Work out the finished part from the listing and answer in its coordinate system (mm). A direction names the side the tool comes from. Give positions to 0.01 mm unless a question says otherwise; leave off trailing zeros. Loops run counter-clockwise (first coordinate to the right, second up) from the corner with the lowest first, then second, coordinate; pieces in that order, holes last. Notation, with made-up numbers: M 9.25,56.25 L 45.25,56.25 A21 cw 45.25,71.25 Z; hole C -37,75.25 d3. An arc over 180 degrees is marked long. Use a Markdown table: item, result.
```python
from build123d import *

# Parameters (mm, degrees)
SKETCH1_W                      = 40.64
SKETCH1_H                      = 2.54
BASE_EXTRUDE_DEPTH             = 5
SKETCH2_W                      = 1.524
SKETCH2_H                      = 0.254
STANDOFF_WIDTH_DEPTH           = 41.966114046
UPPER_START                    = -19.4945
UPPER_CORE_OUTLINE_W           = 3.3528
UPPER_CORE_OUTLINE_H           = 0.889
UPPER_CORE_DEPTH               = 0.889
LEAD_IN_SIZE                   = 0.3937
LEAD_IN_SIZE2                  = 0.469193389
CORE_PATTERN_COUNT             = 16
CORE_PATTERN_PITCH             = 2.54
LEAD_IN_OF_CORE_PATTERN_SIZE2  = 0.469193389
LEAD_IN_OF_CORE_PATTERN_SIZE   = 0.3937
POSITION_CUT_DEPTH             = 21.964620197
SKETCH10_W                     = 0.2794
SKETCH10_H                     = 0.254
STANDOFF_LENGTH_DEPTH          = 22.07970588
STANDOFF_PATTERN_COUNT         = 16
STANDOFF_PATTERN_PITCH         = 2.54
SKETCH11_W                     = 0.635
SKETCH11_H                     = 0.4064
TAIL_DEPTH                     = 3.175
TAIL_FILLETS_R                 = 0.3175
TAIL_PATTERN_COUNT             = 16
TAIL_PATTERN_PITCH             = 2.54
TAIL_FILLETS_OF_TAIL_PATTERN_R = 0.3175
SKETCH12_W                     = 27.94
SKETCH12_H                     = 7.921
CUT_EXTRUDE1_DEPTH             = 22.07970588


# Read off the part's stored shape, not the designer's step: Upper Core
with BuildPart() as part:
    # Sketch1 → Base-Extrude (new body)
    with BuildSketch(Plane(origin=(0, 0, 0), x_dir=(1, 0, 0), z_dir=(0, 1, 0))):
        Rectangle(SKETCH1_W, SKETCH1_H)
    extrude(amount=BASE_EXTRUDE_DEPTH)

    # Sketch2 → Standoff - Width (cut, through all)
    with BuildSketch(Plane.ZY.offset(20.32)):
        with Locations((0, 0.127)):
            Rectangle(SKETCH2_W, SKETCH2_H)
    extrude(amount=-STANDOFF_WIDTH_DEPTH, mode=Mode.SUBTRACT)

    # Upper Core outline → Upper Core (cut)
    with BuildSketch(Plane.YZ.offset(UPPER_START)):
        with Locations((3.3236, 0)):
            Rectangle(UPPER_CORE_OUTLINE_W, UPPER_CORE_OUTLINE_H)
    upper_core = extrude(amount=UPPER_CORE_DEPTH, mode=Mode.SUBTRACT)

    # Lead-in
    lead_in_edges = [part.edges().sort_by_distance(p)[0] for p in [
        (-19.4945, 5, 0),
        (-19.05, 5, 0.4445),
        (-18.6055, 5, 0),
        (-19.05, 5, -0.4445),
    ]]
    lead_in_side = [part.faces().sort_by_distance(p)[0] for p in [
        (0.146976854, 5, 0),
    ]]
    chamfer(lead_in_edges, length=LEAD_IN_SIZE, length2=LEAD_IN_SIZE2, reference=lead_in_side[0])

    # Core Pattern: Upper Core ×16
    with Locations(*[(i * CORE_PATTERN_PITCH, 0, 0) for i in range(1, CORE_PATTERN_COUNT)]):
        add(upper_core, mode=Mode.SUBTRACT)

    # Lead-in of Core Pattern
    lead_in_of_core_pattern_edges = [part.edges().sort_by_distance(p)[0] for p in [
        (-16.9545, 5, 0),
        (-16.51, 5, 0.4445),
        (-16.0655, 5, 0),
        (-16.51, 5, -0.4445),
        (-14.4145, 5, 0),
        (-13.97, 5, 0.4445),
        (-13.5255, 5, 0),
        (-13.97, 5, -0.4445),
        (-11.8745, 5, 0),
        (-11.43, 5, 0.4445),
        (-10.9855, 5, 0),
        (-11.43, 5, -0.4445),
        (-9.3345, 5, 0),
        (-8.89, 5, 0.4445),
        (-8.4455, 5, 0),
        (-8.89, 5, -0.4445),
        (-6.7945, 5, 0),
        (-6.35, 5, 0.4445),
        (-5.9055, 5, 0),
        (-6.35, 5, -0.4445),
        (-4.2545, 5, 0),
        (-3.81, 5, 0.4445),
        (-3.3655, 5, 0),
        (-3.81, 5, -0.4445),
        (-1.7145, 5, 0),
        (-1.27, 5, 0.4445),
        (-0.8255, 5, 0),
        (-1.27, 5, -0.4445),
        (0.8255, 5, 0),
        (1.27, 5, 0.4445),
        (1.7145, 5, 0),
        (1.27, 5, -0.4445),
        (3.3655, 5, 0),
        (3.81, 5, 0.4445),
        (4.2545, 5, 0),
        (3.81, 5, -0.4445),
        (5.9055, 5, 0),
        (6.35, 5, 0.4445),
        (6.7945, 5, 0),
        (6.35, 5, -0.4445),
        (8.4455, 5, 0),
        (8.89, 5, 0.4445),
        (9.3345, 5, 0),
        (8.89, 5, -0.4445),
        (10.9855, 5, 0),
        (11.43, 5, 0.4445),
        (11.8745, 5, 0),
        (11.43, 5, -0.4445),
        (13.5255, 5, 0),
        (13.97, 5, 0.4445),
        (14.4145, 5, 0),
        (13.97, 5, -0.4445),
        (16.0655, 5, 0),
        (16.51, 5, 0.4445),
        (16.9545, 5, 0),
        (16.51, 5, -0.4445),
        (18.6055, 5, 0),
        (19.05, 5, 0.4445),
        (19.4945, 5, 0),
        (19.05, 5, -0.4445),
    ]]
    chamfer(lead_in_of_core_pattern_edges, length=LEAD_IN_OF_CORE_PATTERN_SIZE, length2=LEAD_IN_OF_CORE_PATTERN_SIZE2)

    # Sketch4 → Position Cut (cut, through all)
    with BuildSketch(Plane(origin=(0, 5, 0), x_dir=(-1, 0, 0), z_dir=(0, 1, 0))):
        Polygon((20.32, 1.016), (20.212646968, 1.016), (20.066, 1.27), (20.32, 1.27), align=None)
        Polygon((20.066, -1.27), (20.32, -1.27), (20.32, -1.016), (20.212646968, -1.016), align=None)
        Polygon((17.78, -1.016), (17.887353032, -1.016), (18.034, -1.27), (17.78, -1.27), align=None)
        Polygon((18.034, 1.27), (17.78, 1.27), (17.78, 1.016), (17.887353032, 1.016), align=None)
    position_cut = extrude(amount=-POSITION_CUT_DEPTH, mode=Mode.SUBTRACT)

    # Sketch10 → Standoff - Length (cut, through all)
    with BuildSketch(Plane.XY.offset(1.27)):
        with Locations((-17.9197, 0.127)):
            Rectangle(SKETCH10_W, SKETCH10_H)
        with Locations((-20.1803, 0.127)):
            Rectangle(SKETCH10_W, SKETCH10_H)
    standoff_length = extrude(amount=-STANDOFF_LENGTH_DEPTH, mode=Mode.SUBTRACT)

    # Standoff Pattern: Position Cut, Standoff - Length ×16
    with Locations(*[(i * STANDOFF_PATTERN_PITCH, 0, 0) for i in range(1, STANDOFF_PATTERN_COUNT)]):
        add(position_cut, mode=Mode.SUBTRACT)
        add(standoff_length, mode=Mode.SUBTRACT)

    # Sketch11 → Tail (add)
    with BuildSketch(Plane.XZ.offset(-0.254)):
        with Locations((-19.05, 0)):
            Rectangle(SKETCH11_W, SKETCH11_H)
    tail = extrude(amount=TAIL_DEPTH)

    # Tail Fillets
    tail_fillets_edges = [part.edges().sort_by_distance(p)[0] for p in [
        (-19.3675, -2.921, 0),
        (-18.7325, -2.921, 0),
    ]]
    fillet(tail_fillets_edges, radius=TAIL_FILLETS_R - 0.0001)  # a hair under: the kernel refuses the full size

    # Tail Pattern: Tail ×16
    with Locations(*[(i * TAIL_PATTERN_PITCH, 0, 0) for i in range(1, TAIL_PATTERN_COUNT)]):
        add(tail)

    # Tail Fillets of Tail Pattern
    tail_fillets_of_tail_pattern_edges = [part.edges().sort_by_distance(p)[0] for p in [
        (-16.8275, -2.921, 0),
        (-16.1925, -2.921, 0),
        (-14.2875, -2.921, 0),
        (-13.6525, -2.921, 0),
        (-11.7475, -2.921, 0),
        (-11.1125, -2.921, 0),
        (-9.2075, -2.921, 0),
        (-8.5725, -2.921, 0),
        (-6.6675, -2.921, 0),
        (-6.0325, -2.921, 0),
        (-4.1275, -2.921, 0),
        (-3.4925, -2.921, 0),
        (-1.5875, -2.921, 0),
        (-0.9525, -2.921, 0),
        (0.9525, -2.921, 0),
        (1.5875, -2.921, 0),
        (3.4925, -2.921, 0),
        (4.1275, -2.921, 0),
        (6.0325, -2.921, 0),
        (6.6675, -2.921, 0),
        (8.5725, -2.921, 0),
        (9.2075, -2.921, 0),
        (11.1125, -2.921, 0),
        (11.7475, -2.921, 0),
        (13.6525, -2.921, 0),
        (14.2875, -2.921, 0),
        (16.1925, -2.921, 0),
        (16.8275, -2.921, 0),
        (18.7325, -2.921, 0),
        (19.3675, -2.921, 0),
    ]]
    fillet(tail_fillets_of_tail_pattern_edges, radius=TAIL_FILLETS_OF_TAIL_PATTERN_R - 0.0001)  # a hair under: the kernel refuses the full size

    # Sketch12 → Cut-Extrude1 (cut, through all)
    with BuildSketch(Plane.XY.offset(1.27)):
        with Locations((6.35, 1.0395)):
            Rectangle(SKETCH12_W, SKETCH12_H)
    extrude(amount=-CUT_EXTRUDE1_DEPTH, mode=Mode.SUBTRACT)


solid = part.part
```
(1) The mould has two halves that part along X. Classify faces 3 (the flat face through (-7.62, 3, 0)), 4 (the flat face through (-11.4, 1.647, 0)), 5 (the flat face through (-9, 2, 1.27)): released by +X, released by -X, zero draft, split by the parting line, or undercut.
Entries:
| item | result |
|---|---|
| face 3 | released by +X |
| face 4 | undercut |
| face 5 | zero draft |
(2) A cutting plane is placed at D-D (x = -9.5). Write down the section's boundary in (y, z).
Entries:
| item | result |
|---|---|
| outline | M 0,-1.27 L 5,-1.27 L 5,-0.84 L 4.73,-0.61 L 4.73,0.61 L 5,0.84 L 5,1.27 L 0,1.27 L 0,0.76 L 0.25,0.76 L 0.25,-0.76 L 0,-0.76 Z |
(3) Consider probe 1 along Z at (x, y) = (-11.5, 2.75); probe 2 along Y at (x, z) = (-9.75, 0.05); probe 3 along Y at (x, z) = (-19, 1). Determine where each line is inside the solid, lowest interval first. Write a range as [from, to].
Entries:
| item | result |
|---|---|
| probe 1 | z = [-1.27, -0.44], [0.44, 1.27] |
| probe 2 | y = [0.25, 5] |
| probe 3 | y = [0, 5] |
(4) A cutting plane is placed at C-C (y = 2.5). Count the separate pieces of the cut face and the enclosed holes in it, and give its area (3 significant figures).
Entries:
| item | result |
|---|---|
| separate pieces | 1 |
| enclosed holes | 5 |
| area | 27.4 mm² |
(5) Which of the six approach directions +Z, -Z, +X, -X, +Y, -Y give full straight-line access (tool end or side, diameter ignored) to faces 1 (the flat face through (-8.446, 3, 0)), 2 (the flat face through (-11, 2, -1.27))?
Entries:
| item | result |
|---|---|
| face 1 | +Y |
| face 2 | -Z, +X, -X, +Y, -Y |
(6) A cutting plane is placed at A-A (y = -1.75). Write down the section's boundary in (x, z).
Entries:
| item | result |
|---|---|
| outline | M -19.37,-0.2 L -18.73,-0.2 L -18.73,0.2 L -19.37,0.2 Z; M -16.83,-0.2 L -16.19,-0.2 L -16.19,0.2 L -16.83,0.2 Z; M -14.29,-0.2 L -13.65,-0.2 L -13.65,0.2 L -14.29,0.2 Z; M -11.75,-0.2 L -11.11,-0.2 L -11.11,0.2 L -11.75,0.2 Z; M -9.21,-0.2 L -8.57,-0.2 L -8.57,0.2 L -9.21,0.2 Z |
(7) A cutting plane is placed at B-B (z = 0.6). Write down the section's boundary in (x, y).
Entries:
| item | result |
|---|---|
| outline | M -20.32,0.25 L -7.62,0.25 L -7.62,5 L -8.05,5 L -8.29,4.72 L -9.49,4.72 L -9.73,5 L -10.59,5 L -10.83,4.72 L -12.03,4.72 L -12.27,5 L -13.13,5 L -13.37,4.72 L -14.57,4.72 L -14.81,5 L -15.67,5 L -15.91,4.72 L -17.11,4.72 L -17.35,5 L -18.21,5 L -18.45,4.72 L -19.65,4.72 L -19.89,5 L -20.32,5 Z |
(8) Given P1, Ø1, axis at x = -14, z = 0, coming from the +Y side, flat-ended and moving along its own axis, determine where the tip first touches the part or whether it passes through.
Entries:
| item | result |
|---|---|
| P1 | stops at y = 4.63 |
